Part print with two shaded views. Sizes in mm from the minimum x, y, z corner. Give positions to 0.01 mm unless a question says otherwise; leave off trailing zeros. Write each loop counter-clockwise with the first axis right and the second up, starting at its lowest first coordinate (ties: lowest second). Pieces come first, ordered by that corner, then holes.
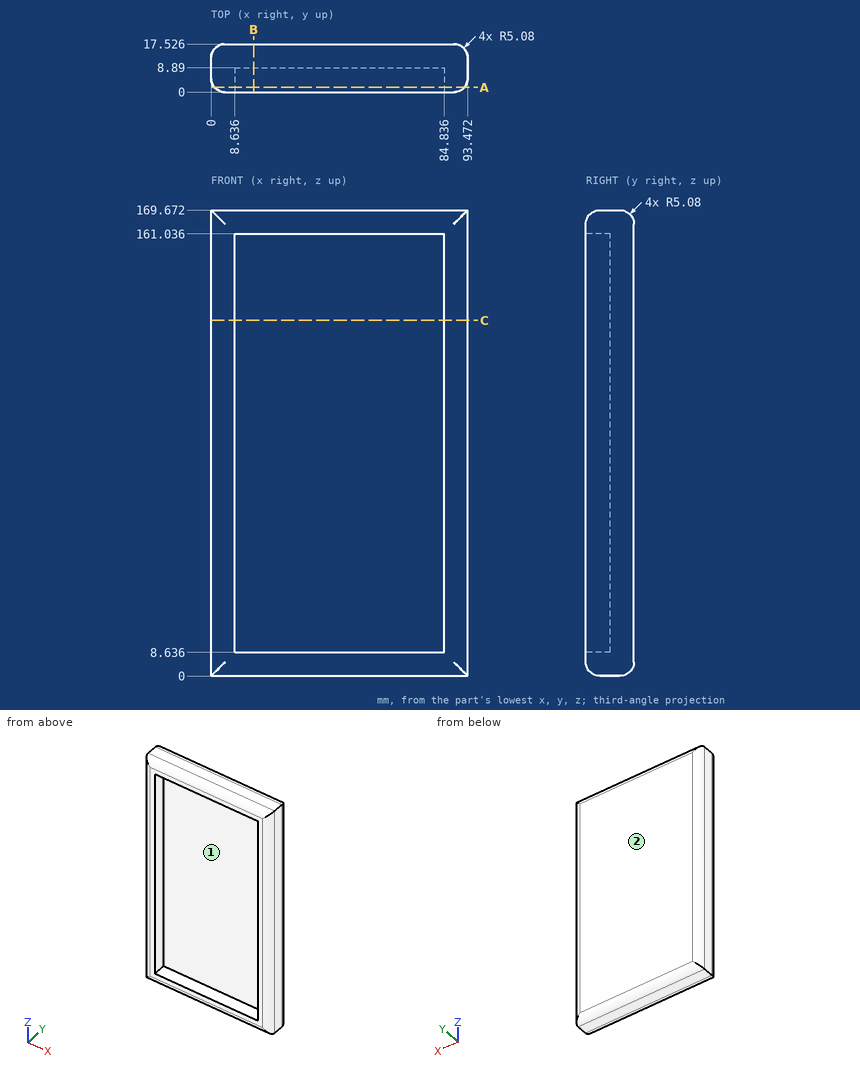
1) Saw through at C-C, the plane z = 129.5. Write the cut outline in (x, y), then the cut area to 3 significant figures.
Answers follow:
outline: (0, 5.08) arc R5.08 ccw to (5.08, 0) - (8.64, 0) - (8.64, 8.89) - (84.84, 8.89) - (84.84, 0) - (88.39, 0) arc R5.08 ccw to (93.47, 5.08) - (93.47, 12.45) arc R5.08 ccw to (88.39, 17.53) - (5.08, 17.53) arc R5.08 ccw to (0, 12.45) - close
area: 939 mm2
2) Saw through at B-B, the plane x = 15.5. Write the cut outline in (y, z).
Answers follow:
outline: (0, 5.08) arc R5.08 ccw to (5.08, 0) - (12.45, 0) arc R5.08 ccw to (17.53, 5.08) - (17.53, 164.59) arc R5.08 ccw to (12.45, 169.67) - (5.08, 169.67) arc R5.08 ccw to (0, 164.59) - (0, 161.04) - (8.89, 161.04) - (8.89, 8.64) - (0, 8.64) - close
3) Two-plate mould, pull along Z, no slides. Class the marked faces 1 and 2: +Z half, -Z half, draft (parallel to the pull), parting line (faces both ways), or undercut.
Answers follow:
face 1: undercut
face 2: draft
4) Pin check, flat tips, straight feed: pin 1 Ø2 at (y, z) = (3.5, 76.5) entering from -X; pin 2 Ø5 at (x, z) = (54.5, 26) entering from -Y; pin 3 Ø2 at (x, y) = (60.5, 3) entering from -Z. Stop position of each tip, or through.
Answers follow:
pin 1: stops at x = 0.03
pin 2: stops at y = 8.89
pin 3: stops at z = 0.12
5) Saw through at A-A, the plane y = 1.75. Write the cut outline in (x, z), then the cut area to 3 significant figures.
Answers follow:
outline: (1.24, 1.24) - (92.23, 1.24) - (92.23, 168.43) - (1.24, 168.43) - close; hole (8.64, 8.64) - (84.84, 8.64) - (84.84, 161.04) - (8.64, 161.04) - close
area: 3,600 mm2
6) Wall check: L1, parallel to Z at x = 59.5, y = 4.5; L2, parallel to Z at x = 53, y = 5.75; L3, parallel to Y at x = 63.5, z = 157. Give the ranges that are in metal, low to high.
Answers follow:
L1: z = 0.03 to 8.64, 161.04 to 169.64
L2: z = 0 to 8.64, 161.04 to 169.67
L3: y = 8.89 to 17.53
